Answer from the drawing. Dimensions are ordinates in mm from the lowest x, y and z of the part. A direction names the side the tool comes from. Round coordinates to 2 decimals unless told otherwise and drop trailing zeros. Loops run counter-clockwise (first coordinate to the right, second up) from the corner with the lowest first, then second, coordinate; pieces in that order, holes last. Notation, with made-up numbers: M 21,31 L 30,31 A20 ccw 30,61 Z; hole C 3,-11.5 d8. An arc over 180 degrees is marked long. Answer as a JSON object with one key per item and string values.
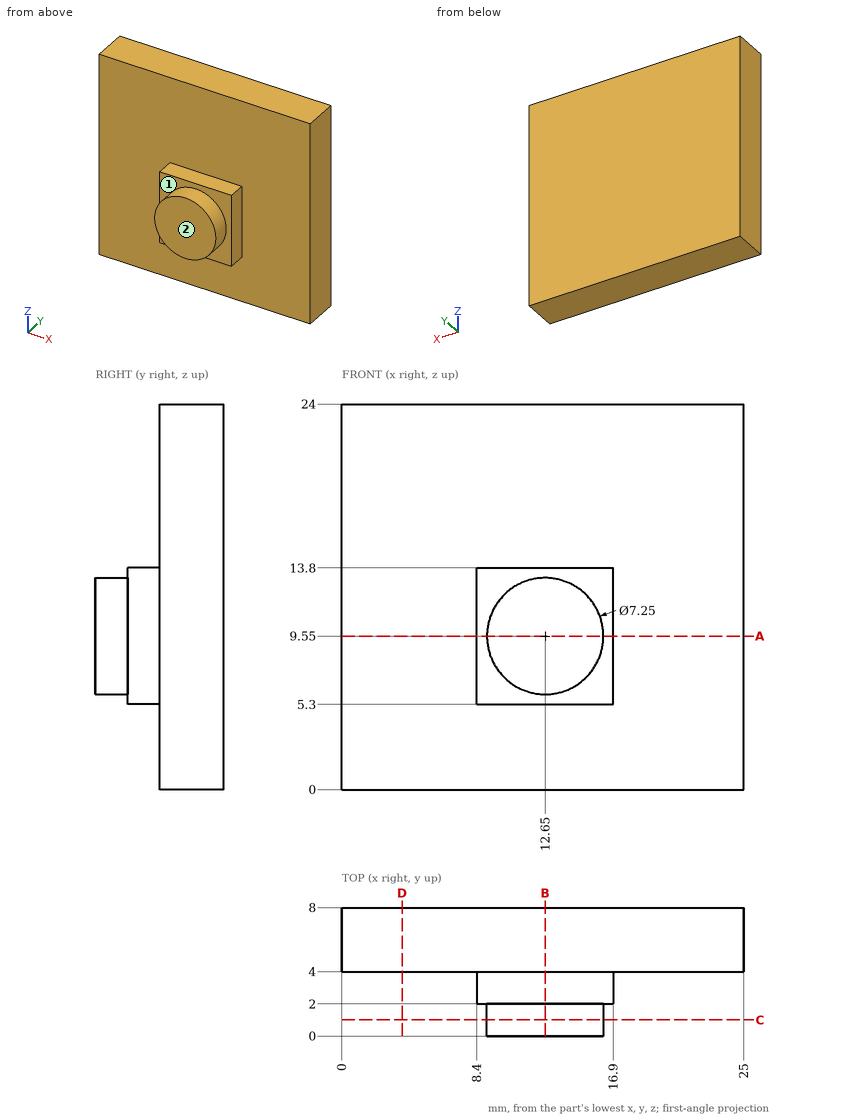
Item 1: The part is cut by section A-A (z = 9.55). Give the vertices of the cut face in (x, y) (3 decimals), then the cut area to 4 significant figures.
Values follow:
{"outline": "M 0,4 L 8.4,4 L 8.4,2 L 9.025,2 L 9.025,0 L 16.275,0 L 16.275,2 L 16.9,2 L 16.9,4 L 25,4 L 25,8 L 0,8 Z", "area": "131.5 mm^2"}
Item 2: The part is cut by section B-B (x = 12.65). Give the vertices of the cut face in (y, z) (3 decimals).
Values follow:
{"outline": "M 0,5.925 L 2,5.925 L 2,5.3 L 4,5.3 L 4,0 L 8,0 L 8,24 L 4,24 L 4,13.8 L 2,13.8 L 2,13.175 L 0,13.175 Z"}
Item 3: The part is cut by section D-D (x = 3.75). Give the vertices of the cut face in (y, z).
Values follow:
{"outline": "M 4,0 L 8,0 L 8,24 L 4,24 Z"}
Item 4: The part is cut by section C-C (y = 1). Give the vertices of the cut face in (x, z) (3 decimals), then the cut area to 3 significant figures.
Values follow:
{"outline": "C 12.65,9.55 d7.25", "area": "41.3 mm^2"}
Item 5: Straight lines are drawn through the part: line 1 (Y direction, x = 21.75, z = 16.25); line 2 (X direction, y = 2.25, z = 7.25); line 3 (X direction, y = 0.5, z = 8.75). For each, find the intervals that lie inside material, in ascending order.
Values follow:
{"line 1": "4 to 8", "line 2": "8.4 to 16.9", "line 3": "9.11 to 16.19"}
Item 6: Which of the six approach directions +Z, -Z, +X, -X, +Y, -Y give full straight-line access (tool end or side, diameter ignored) to the marked faces 1 and 2?
Values follow:
{"face 1": "-Y", "face 2": "+Z, -Z, +X, -X, -Y"}
Item 7: Flat-ended cylindrical pins translate along their axes: P1, Ø2, axis at x = 11, y = 2.5, coming from the -Z side; P2, Ø1.6, axis at y = 3, z = 8, coming from the -X side; P3, Ø12, axis at x = 6, z = 18, coming from the -Y side. Find the tip coordinate at first contact, or state that the pin passes through.
Values follow:
{"P1": "z = 5.3", "P2": "x = 8.4", "P3": "y = 2"}
